from build123d import *

# Parameters (mm, degrees)
BOSS_EXTRUDE4_DEPTH     = 5
SKETCH5_3_R             = 5
BOSS_EXTRUDE5_DEPTH     = 105
FILLET3_R               = 20
SKETCH9_R               = 10
BOSS_EXTRUDE8_DEPTH     = 10
SKETCH5_4_W             = 42
SKETCH5_4_H             = 42
BOSS_EXTRUDE6_DEPTH     = 60
CHAMFER1_SIZE           = 5
SKETCH7_R               = 10
BOSS_EXTRUDE7_DEPTH     = 10
CUT_EXTRUDE2_DEPTH      = 210
CUT_EXTRUDE2_DEPTH_BACK = 10
SKETCH8_R               = 5


with BuildPart() as part:
    # Sketch5 → Boss-Extrude4 (new body)
    with BuildSketch(Plane.XY):
        with BuildLine():
            ThreePointArc((-22.338990751, -25.429636041), (-10.689321102, -51.161900175), (-6.7, -79.125260802))
            Line((-6.7, -79.125260802), (-6.7, -130))
            Line((-6.7, -130), (35.8, -130))
            Line((35.8, -130), (35.8, -50))
            Line((35.8, -50), (32.5, 0))
            ThreePointArc((32.5, 0), (-9.088092204, 31.203470642), (-27.417328006, -17.451078047))
            Line((-27.417328006, -17.451078047), (-22.338990751, -25.429636041))
        make_face()
        with BuildLine():
            ThreePointArc((11.55, -111), (14.55, -110), (17.55, -111))
            Line((17.55, -111), (11.55, -111))
        make_face(mode=Mode.SUBTRACT)
        with BuildLine():
            ThreePointArc((17.857189139, -111.25), (14.55, -120), (11.242810861, -111.25))
            Line((11.242810861, -111.25), (17.857189139, -111.25))
        make_face(mode=Mode.SUBTRACT)
        with BuildLine():
            Line((11.55, -69), (17.55, -69))
            ThreePointArc((17.55, -69), (14.55, -70), (11.55, -69))
        make_face(mode=Mode.SUBTRACT)
        with BuildLine():
            Line((17.857189139, -68.75), (11.242810861, -68.75))
            ThreePointArc((11.242810861, -68.75), (14.55, -60), (17.857189139, -68.75))
        make_face(mode=Mode.SUBTRACT)
    extrude(amount=BOSS_EXTRUDE4_DEPTH)

    # Sketch5<3> → Boss-Extrude5 (add)
    with BuildSketch(Plane.XY):
        with Locations((14.55, -65)):
            Circle(SKETCH5_3_R)
        with Locations((14.55, -115)):
            Circle(SKETCH5_3_R)
    extrude(amount=BOSS_EXTRUDE5_DEPTH)

    # Fillet3
    fillet3_edges = [part.edges().sort_by_distance(p)[0] for p in [
        (35.8, -130, 2.5),
        (-6.7, -130, 2.5),
    ]]
    fillet(fillet3_edges, radius=FILLET3_R)

    # Sketch9 → Boss-Extrude8 (add)
    with BuildSketch(Plane(origin=(0, 0, 0), x_dir=(-1, 0, 0), z_dir=(0, 0, -1))):
        with Locations(Location((0, 0, 0), (0, 0, 180))):
            Circle(SKETCH9_R)
    extrude(amount=BOSS_EXTRUDE8_DEPTH)

    # Mirror3: part across plane


with BuildPart() as part_1:
    add(part.part)
    add(part.part.mirror(Plane(origin=(14.55, -65, 105), x_dir=(1, 0, 0), z_dir=(0, 0, 1))))

    # Sketch5<4> → Boss-Extrude6 (add)
    with BuildSketch(Plane.XY):
        with Locations((14.55, -90)):
            Rectangle(SKETCH5_4_W, SKETCH5_4_H)
    extrude(amount=-BOSS_EXTRUDE6_DEPTH)

    # Chamfer1
    chamfer1_edges = [part_1.edges().sort_by_distance(p)[0] for p in [
        (-6.45, -111, -30),
        (-6.45, -69, -30),
        (35.55, -69, -30),
        (35.55, -111, -30),
    ]]
    chamfer(chamfer1_edges, length=CHAMFER1_SIZE)

    # Sketch7 → Boss-Extrude7 (add)
    with BuildSketch(Plane.XY.offset(210)):
        with Locations(Location((14.55, -90, 0), (0, 0, 180))):
            Circle(SKETCH7_R)
    extrude(amount=BOSS_EXTRUDE7_DEPTH)

    # Sketch8 → Cut-Extrude2 (cut, two sides: drawn at the far end of the back side and taken through both)
    with BuildSketch(Plane.XY.offset(5).offset(-CUT_EXTRUDE2_DEPTH_BACK)):
        with Locations(Location((14.55, -90, 0), (0, 0, 180))):
            Circle(SKETCH8_R)
    extrude(amount=CUT_EXTRUDE2_DEPTH + CUT_EXTRUDE2_DEPTH_BACK, mode=Mode.SUBTRACT)


solid = part_1.part
Verification items for the finished model (mm, model axes). A direction names the side the tool comes from. Coordinates: 2 decimals unless noted, no trailing zeros. Order: outer loops, then holes, each group sorted by start corner. A loop starts at its lowest first (then second) coordinate and runs counter-clockwise, first axis right, second up.
1. Go/stop test with flat-tipped pins: pin 1 Ø2 at (x, y) = (-11.5, 6.5) entering from -Z; pin 2 Ø4 at (y, z) = (-92, 1.5) entering from -X; pin 3 Ø10 at (x, y) = (2, -0.5) entering from -Z; pin 4 Ø1.5 at (x, z) = (-8.5, -18) entering from +Y. Record where each tip stops, or that it passes through.
Results found:
pin 1: stops at z = 0
pin 2: stops at x = -6.7
pin 3: stops at z = -10
pin 4: passes through
2. Release check for a two-part mould opening along Z. For faces 6 (the face through (-3.985, -108.465, -29.58)), 7 (the face through (15, -90, 220)), 8 (the face through (15.63, -85.12, 209.93)) record: +Z half, -Z half, draft (parallel to the pull), parting line (faces both ways), or undercut.
Results found:
face 6: draft
face 7: +Z half
face 8: undercut
3. Sectioned sample at C-C, the plane z = -20. Record the cut outline in (x, y), and give its area (3 significant figures).
Results found:
outline: (-6.45, -106) - (-1.45, -111) - (30.55, -111) - (35.55, -106) - (35.55, -74) - (30.55, -69) - (-1.45, -69) - (-6.45, -74) - close
area: 1,710 mm2
4. Sectioned sample at D-D, the plane y = -65. Record the cut outline in (x, z), and give its area (3 significant figures).
Results found:
outline: (-7.7, 0) - (35.8, 0) - (35.8, 5) - (19.55, 5) - (19.55, 205) - (35.8, 205) - (35.8, 210) - (-7.7, 210) - (-7.7, 205) - (9.55, 205) - (9.55, 5) - (-7.7, 5) - close
area: 2,440 mm2
5. Set-up check for faces 1 (the face through (15.63, -85.12, -0.07)), 2 (the face through (33.085, -108.465, -29.58)), 3 (the face through (0, 0, -10)), 4 (the face through (-10, 0, 215)), 5 (the face through (35.55, -90, -30)): record each of +Z, -Z, +X, -X, +Y, -Y from which the full face is reachable in a straight line by a thin tool's end or side.
Results found:
face 1: none
face 2: -Z, +X, -Y
face 3: -Z, +X, -X, +Y
face 4: +Z
face 5: -Z, +X, +Y, -Y
6. Scan lines: line 1 (X direction, y = -90, z = 207); line 2 (Y direction, x = 14.55, z = -1.5); line 3 (Z direction, x = -1, y = -84). Record each from-to range of solid material in increasing order.
Results found:
line 1: x = -6.7 to 9.55, 19.55 to 35.8
line 2: y = -111 to -95, -85 to -69
line 3: z = -60 to 5, 205 to 210
7. Sectioned sample at B-B, the plane z = 13. Record the cut outline in (x, y).
Results found:
outline: circle Ø10 at (14.55, -115); circle Ø10 at (14.55, -65)
8. Sectioned sample at A-A, the plane y = -90. Record the cut outline in (x, z), and give its area (4 significant figures).
Results found:
outline: (-6.7, 0) - (-6.45, 0) - (-6.45, -60) - (35.55, -60) - (35.55, 0) - (35.8, 0) - (35.8, 5) - (19.55, 5) - (19.55, -5) - (9.55, -5) - (9.55, 5) - (-6.7, 5) - close; (-6.7, 205) - (9.55, 205) - (9.55, 215) - (19.55, 215) - (19.55, 205) - (35.8, 205) - (35.8, 210) - (24.55, 210) - (24.55, 220) - (4.55, 220) - (4.55, 210) - (-6.7, 210) - close
area: 2,945 mm2
